from build123d import *

# Parameters (mm, degrees)
SKETCH2_W           = 150
SKETCH2_H           = 80
SKETCH3_R           = 15
BOSS_EXTRUDE1_DEPTH = 10


with BuildPart() as part:
    # Sketch2 → Loft1 section 0
    with BuildSketch(Plane(origin=(100, 0, 0), x_dir=(0, 0, -1), z_dir=(1, 0, 0))):
        Rectangle(SKETCH2_W, SKETCH2_H)
    # Sketch1 for Loft1 → Loft1 section 1
    with BuildSketch(Plane(origin=(0, 0, 0), x_dir=(0, 0, -1), z_dir=(1, 0, 0))):
        with BuildLine():
            # circular arc as an exact rational Bezier (weights 1, cos(half-angle), 1)
            Bezier((-22.058823529, 11.764705882), (0, 53.125000003), (22.058823529, 11.764705882), weights=[1, 0.470588235, 1])
            Bezier((22.058823529, 11.764705882), (28.333333334, 0), (22.058823529, -11.764705882), weights=[1, 0.882352941, 1])
            Bezier((22.058823529, -11.764705882), (0, -53.125000003), (-22.058823529, -11.764705882), weights=[1, 0.470588235, 1])
            Bezier((-22.058823529, -11.764705882), (-28.333333334, 0), (-22.058823529, 11.764705882), weights=[1, 0.882352941, 1])
        make_face()
    loft()

    # Sketch3 → Boss-Extrude1 (add)
    with BuildSketch(Plane(origin=(100, 0, 0), x_dir=(0, 0, -1), z_dir=(1, 0, 0))):
        Circle(SKETCH3_R)
    extrude(amount=BOSS_EXTRUDE1_DEPTH)


solid = part.part
Geometry check sheet. Reference: the model listing, model coordinates, mm. A direction names the side the tool comes from. Coordinates: 2 decimals unless noted, no trailing zeros. One line per question, with ' | ' between items.
1. Thickness scan on probe 1 along X at (y, z) = (5, -21); probe 2 along Y at (x, z) = (71, 8); probe 3 along Z at (x, y) = (52, -20). Record the ranges inside material, lowest first. Write a range as from..to.
Answers:
probe 1: x = 0..100 | probe 2: y = -35.56..35.56 | probe 3: z = -50.18..50.18
2. Depth check by flat-ended pin: pin 1 Ø4 at (x, y) = (30.5, -8) entering from -Z; pin 2 Ø1 at (x, z) = (91.5, 43.5) entering from -Y; pin 3 Ø2 at (y, z) = (11, 46) entering from +X. Enter the tip coordinate at first touch or a pass-through.
Answers:
pin 1: stops at z = -40.97 | pin 2: stops at y = -38.33 | pin 3: stops at x = 100
3. Set-up check for faces 1 (the cylindrical face through (104.93, 0.66, 14.985)), 2 (the flat face through (0, -1, 0)): record each of +Z, -Z, +X, -X, +Y, -Y from which the full face is reachable in a straight line by a thin tool's end or side.
Answers:
face 1: +X | face 2: +Z, -Z, -X, +Y, -Y
